```python
from build123d import *

# Parameters (mm, degrees)
SKETCH1_R           = 10.922
SKETCH1_W           = 21.844
SKETCH1_H           = 21.844
BOSS_EXTRUDE1_DEPTH = 22.225
SKETCH2_R           = 7.9375
SKETCH2_W           = 21.844
SKETCH2_H           = 21.844
BOSS_EXTRUDE2_DEPTH = 571.5
BOSS_EXTRUDE3_START = 22.225
SKETCH3_R           = 10.922
SKETCH3_R_2         = 7.9375
BOSS_EXTRUDE3_DEPTH = 22.225


with BuildPart() as part:
    # Sketch1 → Boss-Extrude1 (new body)
    with BuildSketch(Plane.XY):
        with BuildLine():
            Line((0, 9.398), (0, 0))
            Line((0, 0), (5.357138816, 0))
            ThreePointArc((5.357138816, 0), (1.433335767, 3.989179882), (0, 9.398))
        make_face()
        with BuildLine():
            ThreePointArc((0, 9.398), (1.433335767, 3.989179882), (5.357138816, 0))
            Line((5.357138816, 0), (10.922, 0))
            Line((10.922, 0), (10.922, 9.398))
            Line((10.922, 9.398), (10.922, 20.32))
            ThreePointArc((10.922, 20.32), (3.198979736, 17.121020264), (0, 9.398))
        make_face()
        with BuildLine():
            Line((10.922, 9.398), (10.922, 0))
            Line((10.922, 0), (16.486861184, 0))
            ThreePointArc((16.486861184, 0), (20.410664233, 3.989179882), (21.844, 9.398))
            ThreePointArc((21.844, 9.398), (18.645020264, 17.121020264), (10.922, 20.32))
            Line((10.922, 20.32), (10.922, 9.398))
        make_face()
        with BuildLine():
            ThreePointArc((21.844, 9.398), (20.410664233, 3.989179882), (16.486861184, 0))
            Line((16.486861184, 0), (21.844, 0))
            Line((21.844, 0), (21.844, 9.398))
        make_face()
        with BuildLine():
            Line((10.922, 0), (5.357138816, 0))
            ThreePointArc((5.357138816, 0), (10.922, -1.524), (16.486861184, 0))
            Line((16.486861184, 0), (10.922, 0))
        make_face()
        with Locations((10.922, 9.398)):
            Circle(SKETCH1_R)
        with Locations((10.922, -10.922)):
            Rectangle(SKETCH1_W, SKETCH1_H)
    extrude(amount=BOSS_EXTRUDE1_DEPTH)

    # Sketch2 → Boss-Extrude2 (add)
    with BuildSketch(Plane(origin=(0, 0, 0), x_dir=(-1, 0, 0), z_dir=(0, 0, -1))):
        with Locations(Location((-10.922, 9.398, 0), (0, 0, 180))):
            Circle(SKETCH2_R)
        with Locations((-10.922, -10.922)):
            Rectangle(SKETCH2_W, SKETCH2_H)
    boss_extrude2 = extrude(amount=BOSS_EXTRUDE2_DEPTH)

    # Mirror1: Boss-Extrude2 across plane
    add(boss_extrude2.mirror(Plane.XY.offset(-571.5)))

    # Sketch3 → Boss-Extrude3 (add)
    # profile 1 of 3: a face of its own
    with BuildSketch(Plane(origin=(0, 0, -1143), x_dir=(-1, 0, 0), z_dir=(0, 0, -1)).offset(BOSS_EXTRUDE3_START)):
        with BuildLine():
            Line((-21.844, -21.844), (0, -21.844))
            Line((0, -21.844), (0, 9.398))
            ThreePointArc((0, 9.398), (-10.922, -1.524), (-21.844, 9.398))
            Line((-21.844, 9.398), (-21.844, -21.844))
        make_face()
    # profile 2 of 3: a face of its own
    with BuildSketch(Plane(origin=(0, 0, -1143), x_dir=(-1, 0, 0), z_dir=(0, 0, -1)).offset(BOSS_EXTRUDE3_START)):
        with Locations((-10.922, 9.398)):
            Circle(SKETCH3_R)
        with Locations(Location((-10.922, 9.398, 0), (0, 0, 180))):
            Circle(SKETCH3_R_2, mode=Mode.SUBTRACT)
    # profile 3 of 3: a face of its own
    with BuildSketch(Plane(origin=(0, 0, -1143), x_dir=(-1, 0, 0), z_dir=(0, 0, -1)).offset(BOSS_EXTRUDE3_START)):
        with Locations(Location((-10.922, 9.398, 0), (0, 0, 180))):
            Circle(SKETCH3_R_2)
    extrude(amount=-BOSS_EXTRUDE3_DEPTH)


solid = part.part
```
CAD build for the part. Positions are in the model's coordinates, mm. A direction names the side the tool comes from. Round coordinates to 2 decimals unless told otherwise and drop trailing zeros. Write each loop counter-clockwise with the first axis right and the second up, starting at its lowest first coordinate (ties: lowest second). Pieces come first, ordered by that corner, then holes. Notation, with made-up numbers: (40.5, 62) - (81.5, 62) arc R32 ccw to (81.5, 96) - close; hole circle Ø3 at (5, -33.5). An arc over 180 degrees is marked (long way). Write item = value, one per line. Start each with the question number.
Q1. Band-saw the part on B-B (x = 7). Give the cut face in (y, z) (3 decimals), then the cut area to 3 significant figures.
Q2. Probe L1, parallel to Y at x = 11.5, z = -454; L2, parallel to Z at x = 4.5, y = 16 (3 decimals); L3, parallel to Y at x = 18, z = -968.5. List the from-to ranges inside material, lowest first. Write a range as from..to.
Q3. Mould opens along Y. For faces 3 (the flat face through (11, 0, 22.225)), 4 (the flat face through (11, 1, -1143)), 5 (the flat face through (11, -21.844, -580)), 6 (the flat face through (11, 0, -580)) say: pulls with the +Y half, pulls with the -Y half, needs draft (parallel to the pull), parting line crosses it, or undercut.
Q4. Band-saw the part on A-A (z = -723.5). Give the cut face in (x, y) (1 decimal), then the cut area to 3 significant figures.
Q5. Which spindle directions (+Z, -Z, +X, -X, +Y, -Y) get a long thin tool onto all of the face, cutting with end or side? Do faces 1 (the flat face through (11, 1, 0)), 2 (the flat face through (11, 0, -1165.225)). Say none if no direction does.
Q6. Drop flat-ended pins along their axis: pin 1 (8 mm diameter, centred on y = 10, z = -987.5, fed in from +X); pin 2 (5 mm diameter, centred on x = 11, z = -715, fed in from +Y); pin 3 (4 mm diameter, centred on x = 3.5, z = -181.5, fed in from +Y). Give the stop position or say it passes through.
Answers below:
q1.outline = (-21.844, -1165.225) - (19.592, -1165.225) - (19.592, -1143) - (16.299, -1143) - (16.299, 0) - (19.592, 0) - (19.592, 22.225) - (-21.844, 22.225) - close; hole (0, -1143) - (2.497, -1143) - (2.497, 0) - (0, 0) - close
q1.area = 42,600 mm2
q2.L1 = -21.84..0, 1.48..17.31
q2.L2 = -1165.225..-1143, 0..22.225
q2.L3 = -21.84..0, 5.81..12.99
q3.face_3 = needs draft
q3.face_4 = undercut
q3.face_5 = pulls with the -Y half
q3.face_6 = undercut
q4.outline = (0, -21.8) - (21.8, -21.8) - (21.8, 0) - (0, 0) - close; circle Ø15.9 at (10.9, 9.4)
q4.area = 675 mm2
q5.face_1 = none
q5.face_2 = -Z, +X, -X, +Y, -Y
q6.pin_1 = 18.86
q6.pin_2 = 17.34
q6.pin_3 = 15.2
